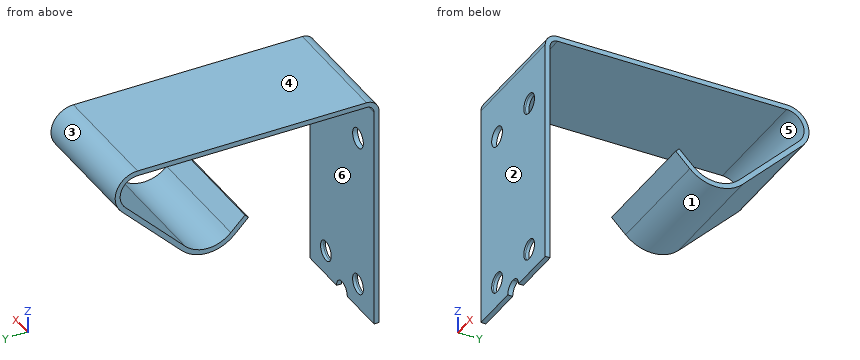
```python
from build123d import *

# Parameters (mm, degrees)
SKETCH002_W       = 6
SKETCH002_H       = 0.25
SKETCH003_R       = 0.5
POCKET_DEPTH      = 5
POCKET_DEPTH_BACK = 5


with BuildPart() as part:
    # AdditivePipe: sweep along a path in Sketch
    with BuildLine(Plane.YZ) as additivepipe_path:
        Line((-1.944544, -0.53033), (-1.237437, -1.237437))
        ThreePointArc((-1.237437, -1.237437), (0, -1.75), (1.237437, -1.237437))
        Line((1.237437, -1.237437), (4.242641, 1.767767))
        ThreePointArc((4.242641, 1.767767), (4.459413, 2.857557), (3.535534, 3.474874))
        Line((3.535534, 3.474874), (-7.964466, 3.474874))
        ThreePointArc((-7.964466, 3.474874), (-8.318019, 3.328427), (-8.464466, 2.974874))
        Line((-8.464466, 2.974874), (-8.464466, -8.275126))
    # Sketch002 (on DatumPlane) → AdditivePipe (sweep)
    with BuildSketch(Plane.XY.offset(-8)):
        with Locations((0, -8.464466)):
            Rectangle(SKETCH002_W, SKETCH002_H)
    sweep(path=additivepipe_path.line)

    # Sketch003 (on DatumPlane) → Pocket (cut, two sides)
    with BuildSketch(Plane.XZ.offset(8.5)) as pocket_sk:
        with Locations((1.5, -7.025126)):
            Circle(SKETCH003_R)
        with Locations((1.5, 0.724874)):
            Circle(SKETCH003_R)
        with BuildLine():
            Line((0, -8.275126), (0, -7.775126))
            ThreePointArc((0.5, -8.275126), (0.353553, -7.921573), (0, -7.775126))
            Line((0, -8.275126), (0.5, -8.275126))
        make_face()
    pocket = extrude(amount=POCKET_DEPTH, mode=Mode.SUBTRACT) + extrude(pocket_sk.sketch, amount=-POCKET_DEPTH_BACK, mode=Mode.SUBTRACT)

    # Mirrored: Pocket across Sketch003 V_Axis
    add(pocket.mirror(Plane(origin=(0, -8.5, 0), x_dir=(0, -1, 0), z_dir=(1, 0, 0))), mode=Mode.SUBTRACT)


solid = part.part
```
Read the model definition and answer for the solid it produces. Units are mm, in the model's axes. Face numbers are marked on the shaded views. A direction names the side the tool comes from. Round coordinates to 2 decimals unless told otherwise and drop trailing zeros. Write each loop counter-clockwise with the first axis right and the second up, starting at its lowest first coordinate (ties: lowest second). Pieces come first, ordered by that corner, then holes. Notation, with made-up numbers: (-28.75, 61) - (-5.75, 61) arc R16 cw to (-5.75, 65) - close; hole circle Ø2 at (59, 64). An arc over 180 degrees is marked (long way). One line per item, written item: value.
Q1. Straight lines are drawn through the part: line 1 (Z direction, x = -1.5, y = -8.5); line 2 (Z direction, x = 1, y = -7.25); line 3 (Y direction, x = -1.25, z = -4.75). For each, find the intervals that lie inside material, in ascending order. Write a range as from..to.
The answers:
line 1: z = -8.28..-7.53, -6.53..0.22, 1.22..3.3
line 2: z = 3.35..3.6
line 3: y = -8.59..-8.34
Q2. Which of the six approach directions +Z, -Z, +X, -X, +Y, -Y give full straight-line access (tool end or side, diameter ignored) to the marked faces 4, 5 and 6?
The answers:
face 4: +Z, +X, -X, +Y, -Y
face 5: +X, -X
face 6: -Z, +X, -X
Q3. For a pull along Y with two mould halves and no side action, classify the marked faces 1, 2 and 3 as pulls with the +Y half, pulls with the -Y half, needs draft (parallel to the pull), parting line crosses it, or undercut.
The answers:
face 1: undercut
face 2: pulls with the -Y half
face 3: pulls with the +Y half
Q4. Each of these flat-tipped pins is pushed along its axis until it touches: P1, Ø1.8, axis at x = -1, z = -3.5, coming from the +Y side; P2, Ø2, axis at x = 2, z = -2, coming from the +Y side; P3, Ø1, axis at x = 1, z = 0, coming from the +Y side. Where does it stop, or does it pass through?
The answers:
P1: stops at y = -8.34
P2: stops at y = 1.65
P3: stops at y = 3.15
Q5. Find section D-D (x = -2.25). Determine the outline of the cut face in (y, z) (3 decimals).
The answers:
outline: (-8.589, -8.275) - (-8.339, -8.275) - (-8.339, 2.975) arc R0.375 cw to (-7.964, 3.35) - (3.536, 3.35) arc R0.875 cw to (4.154, 1.856) - (1.149, -1.149) arc R1.625 cw to (-1.149, -1.149) - (-1.856, -0.442) - (-2.033, -0.619) - (-1.326, -1.326) arc R1.875 ccw to (1.326, -1.326) - (4.331, 1.679) arc R1.125 ccw to (3.536, 3.6) - (-7.964, 3.6) arc R0.625 ccw to (-8.589, 2.975) - close
Q6. Find section C-C (z = -0.25). Determine the outline of the cut face in (x, y), and give its area (3 significant figures).
The answers:
outline: (-3, -8.59) - (3, -8.59) - (3, -8.34) - (-3, -8.34) - close; (-3, 2.05) - (3, 2.05) - (3, 2.4) - (-3, 2.4) - close
area: 3.62 mm2
Q7. Find section B-B (y = 0.75). Determine the outline of the cut face in (x, z).
The answers:
outline: (-3, -1.72) - (3, -1.72) - (3, -1.44) - (-3, -1.44) - close; (-3, 3.35) - (3, 3.35) - (3, 3.6) - (-3, 3.6) - close
Q8. Find section A-A (x = -1.5). Determine the outline of the cut face in (y, z) (3 decimals), and give its area (3 significant figures).
The answers:
outline: (-8.589, -8.275) - (-8.339, -8.275) - (-8.339, -7.525) - (-8.589, -7.525) - close; (-8.589, -6.525) - (-8.339, -6.525) - (-8.339, 0.225) - (-8.589, 0.225) - close; (-8.589, 1.225) - (-8.339, 1.225) - (-8.339, 2.975) arc R0.375 cw to (-7.964, 3.35) - (3.536, 3.35) arc R0.875 cw to (4.154, 1.856) - (1.149, -1.149) arc R1.625 cw to (-1.149, -1.149) - (-1.856, -0.442) - (-2.033, -0.619) - (-1.326, -1.326) arc R1.875 ccw to (1.326, -1.326) - (4.331, 1.679) arc R1.125 ccw to (3.536, 3.6) - (-7.964, 3.6) arc R0.625 ccw to (-8.589, 2.975) - close
area: 7.97 mm2
